from build123d import *

# Parameters (mm, degrees)
ESBO_O1_R                  = 8.5
ESBO_O1_R_2                = 6.5
RESSALTO_EXTRUS_O1_DEPTH   = 3
ESBO_O3_R                  = 7.5
ESBO_O3_R_2                = 6.5
RESSALTO_EXTRUS_O3_DEPTH   = 30
ESBO_O4_R                  = 2
CORTE_EXTRUS_O1_DEPTH      = 9.5
CORTE_EXTRUS_O1_DEPTH_BACK = 9.5


with BuildPart() as part:
    # Esboço1 → Ressalto-extrusão1 (new body)
    with BuildSketch(Plane.XY):
        Circle(ESBO_O1_R)
        Circle(ESBO_O1_R_2, mode=Mode.SUBTRACT)
    extrude(amount=RESSALTO_EXTRUS_O1_DEPTH)

    # Esboço3 → Ressalto-extrusão3 (add)
    with BuildSketch(Plane(origin=(0, 0, 0), x_dir=(-1, 0, 0), z_dir=(0, 0, -1))):
        Circle(ESBO_O3_R)
        Circle(ESBO_O3_R_2, mode=Mode.SUBTRACT)
    extrude(amount=RESSALTO_EXTRUS_O3_DEPTH)

    # Esboço4 → Corte-extrusão1 (cut, two sides)
    with BuildSketch(Plane(origin=(0, 0, 0), x_dir=(0, 0, -1), z_dir=(1, 0, 0))) as corte_extrus_o1_sk:
        with Locations((26, 0)):
            Circle(ESBO_O4_R)
    extrude(amount=CORTE_EXTRUS_O1_DEPTH, mode=Mode.SUBTRACT)
    extrude(corte_extrus_o1_sk.sketch, amount=-CORTE_EXTRUS_O1_DEPTH_BACK, mode=Mode.SUBTRACT)


solid = part.part
Geometry check sheet. Reference: the model listing, model coordinates, mm. A direction names the side the tool comes from. Give positions to 0.01 mm unless a question says otherwise; leave off trailing zeros. Order: outer loops, then holes, each group sorted by start corner. A loop starts at its lowest first (then second) coordinate and runs counter-clockwise, first axis right, second up. Notation, with made-up numbers: M 72.5,46 L 119.5,46 A8 cw 119.5,55 Z; hole C 60.25,80.5 d8. An arc over 180 degrees is marked long. Use a Markdown table: item, result.
Item 1: Section check B-B (y = 0). Record the cut outline in (x, z).
Answers follow:
| item | result |
|---|---|
| outline | M -8.5,0 L -7.5,0 L -7.5,-24 L -6.5,-24 L -6.5,3 L -8.5,3 Z; M -7.5,-30 L -6.5,-30 L -6.5,-28 L -7.5,-28 Z; M 6.5,-30 L 7.5,-30 L 7.5,-28 L 6.5,-28 Z; M 6.5,-24 L 7.5,-24 L 7.5,0 L 8.5,0 L 8.5,3 L 6.5,3 Z |
Item 2: Section check C-C (z = -22.5). Record the cut outline in (x, y), and give its area (3 significant figures).
Answers follow:
| item | result |
|---|---|
| outline | C 0,0 d15; hole C 0,0 d13 |
| area | 44.0 mm2 |
Item 3: Draft check along Y on faces 1 (the flat face through (4.4, -5, 3)), 2 (the cylindrical face through (-6.8, -1.2, -24.4)), 3 (the cylindrical face through (6.8, -1.2, -24.4)), 4 (the cylindrical face through (4.57, 7.167, 1.479)). Enter one of: +Y half, -Y half, draft (parallel to the pull), parting line (faces both ways), or undercut.
Answers follow:
| item | result |
|---|---|
| face 1 | draft |
| face 2 | undercut |
| face 3 | undercut |
| face 4 | parting line |
Item 4: Material ranges on line 1 along X through (y, z) = (-0.25, -5); line 2 along X through (y, z) = (-4.25, -13), recorded low to high.
Answers follow:
| item | result |
|---|---|
| line 1 | x = -7.5 to -6.5, 6.5 to 7.5 |
| line 2 | x = -6.18 to -4.92, 4.92 to 6.18 |
Item 5: Section check A-A (x = 0). Record the cut outline in (y, z), and give its area (3 significant figures).
Answers follow:
| item | result |
|---|---|
| outline | M -8.5,0 L -7.5,0 L -7.5,-30 L -6.5,-30 L -6.5,3 L -8.5,3 Z; M 6.5,-30 L 7.5,-30 L 7.5,0 L 8.5,0 L 8.5,3 L 6.5,3 Z |
| area | 72.0 mm2 |
Item 6: Section check D-D (x = 7). Record the cut outline in (y, z), and give its area (3 significant figures).
Answers follow:
| item | result |
|---|---|
| outline | M -4.82,0 L -2.69,0 L -2.69,-30 L 2.69,-30 L 2.69,0 L 4.82,0 L 4.82,3 L -4.82,3 Z; hole C 0,-26 d4 |
| area | 178 mm2 |
Item 7: Depth check by flat-ended pin: P1, Ø10, axis at x = 6.5, z = -22.5, coming from the +Y side; P2, Ø6, axis at x = 0.5, y = -2.5, coming from the -Z side; P3, Ø5, axis at y = 0, z = -26, coming from the -X side; P4, Ø6, axis at x = 4.5, z = -11.5, coming from the -Y side. Enter the tip coordinate at first touch or a pass-through.
Answers follow:
| item | result |
|---|---|
| P1 | stops at y = 7.35 |
| P2 | passes through |
| P3 | stops at x = -7.5 |
| P4 | stops at y = -7.35 |
Item 8: Tool access check on faces 5 (the flat face through (6, 3, -30)), 6 (the cylindrical face through (-6.93, -2.87, -14.79)). Record the directions out of +Z, -Z, +X, -X, +Y, -Y that give a thin tool (end or side, any length) a straight path to the whole face; none if there is none.
Answers follow:
| item | result |
|---|---|
| face 5 | -Z, +X, -X, +Y, -Y |
| face 6 | -Z |
